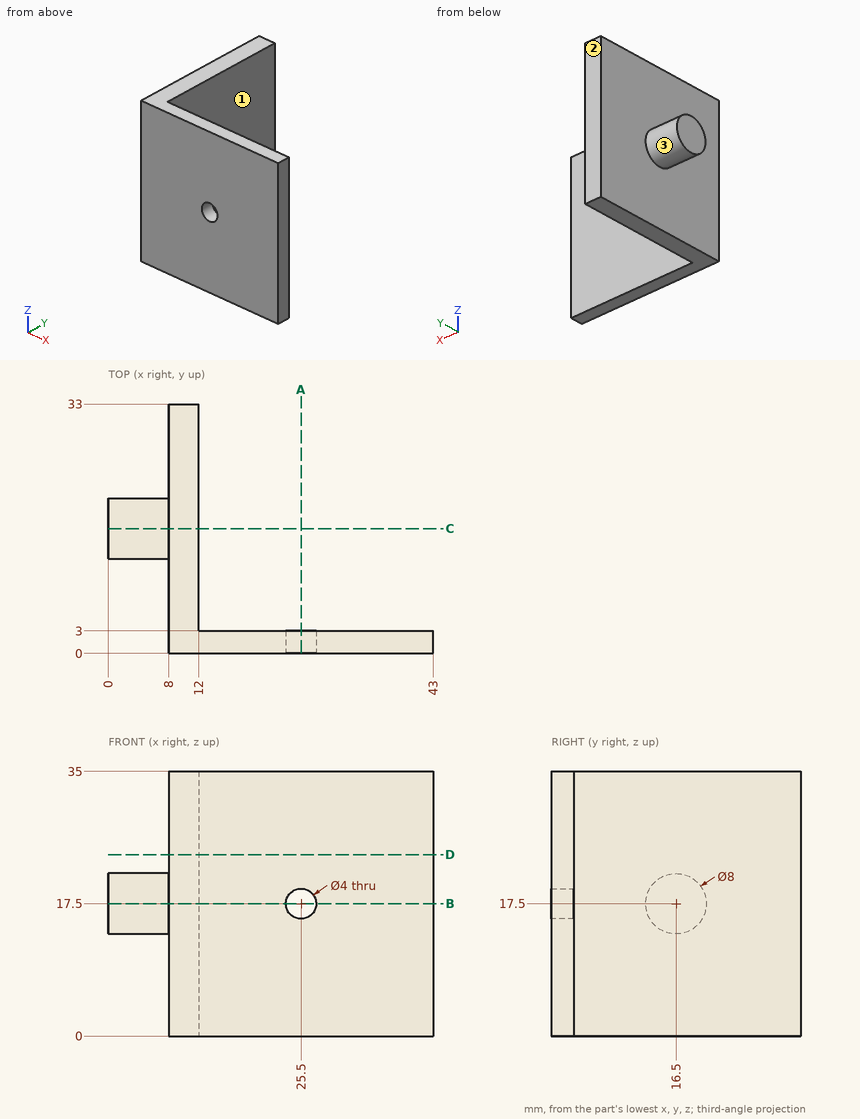
Input: dimensioned drawing with shaded views. Units: mm. Origin: part minimum x, y, z. A direction names the side the tool comes from. Round coordinates to 2 decimals unless told otherwise and drop trailing zeros. Write each loop counter-clockwise with the first axis right and the second up, starting at its lowest first coordinate (ties: lowest second). Pieces come first, ordered by that corner, then holes. Notation, with made-up numbers: (-24.5, -21.75) - (-17.5, -21.75) arc R13 ccw to (-17.5, -8.75) - close; hole circle Ø3 at (-19.5, -38.75). An arc over 180 degrees is marked (long way). Write item = value, one per line.
(1) Section query A-A on x = 25.5. Output: boundary loops of the cut face in (y, z), then the cut area to 3 significant figures.
Geometry check:
outline = (0, 0) - (3, 0) - (3, 15.5) - (0, 15.5) - close; (0, 19.5) - (3, 19.5) - (3, 35) - (0, 35) - close
area = 93.0 mm^2
(2) Material intervals for probe 1 along X at (y, z) = (1.75, 17.5); probe 2 along X at (y, z) = (25, 13); probe 3 along Y at (x, z) = (18.5, 16.5), sorted ascending.
Geometry check:
probe_1 = 8 to 23.5, 27.5 to 43
probe_2 = 8 to 12
probe_3 = 0 to 3
(3) Section query B-B on z = 17.5. Output: boundary loops of the cut face in (x, y), then the cut area to 3 significant figures.
Geometry check:
outline = (0, 12.5) - (8, 12.5) - (8, 0) - (23.5, 0) - (23.5, 3) - (12, 3) - (12, 33) - (8, 33) - (8, 20.5) - (0, 20.5) - close; (27.5, 0) - (43, 0) - (43, 3) - (27.5, 3) - close
area = 277 mm^2
(4) Access query for the marked faces 1, 2 and 3. Directions: +Z, -Z, +X, -X, +Y, -Y. A direction counts if a zero-diameter tool reaches every point of the face in a straight line with its end or side. Return the directions, or none.
Geometry check:
face_1 = +Z, -Z, +X, +Y
face_2 = +Z, -Z, +X, -X, +Y
face_3 = -X
(5) Section query D-D on z = 24. Output: boundary loops of the cut face in (x, y).
Geometry check:
outline = (8, 0) - (43, 0) - (43, 3) - (12, 3) - (12, 33) - (8, 33) - close
(6) Section query C-C on y = 16.5. Output: boundary loops of the cut face in (x, z).
Geometry check:
outline = (0, 13.5) - (8, 13.5) - (8, 0) - (12, 0) - (12, 35) - (8, 35) - (8, 21.5) - (0, 21.5) - close
(7) Contact query for flat-ended pins moving along their axis: pin 1 Ø5 at (y, z) = (22.5, 16) entering from +X; pin 2 Ø1 at (y, z) = (28, 12.5) entering from -X; pin 3 Ø1 at (x, z) = (13, 24.5) entering from +Y. Output: stop coordinate, or through.
Geometry check:
pin_1 = 12
pin_2 = 8
pin_3 = 3
